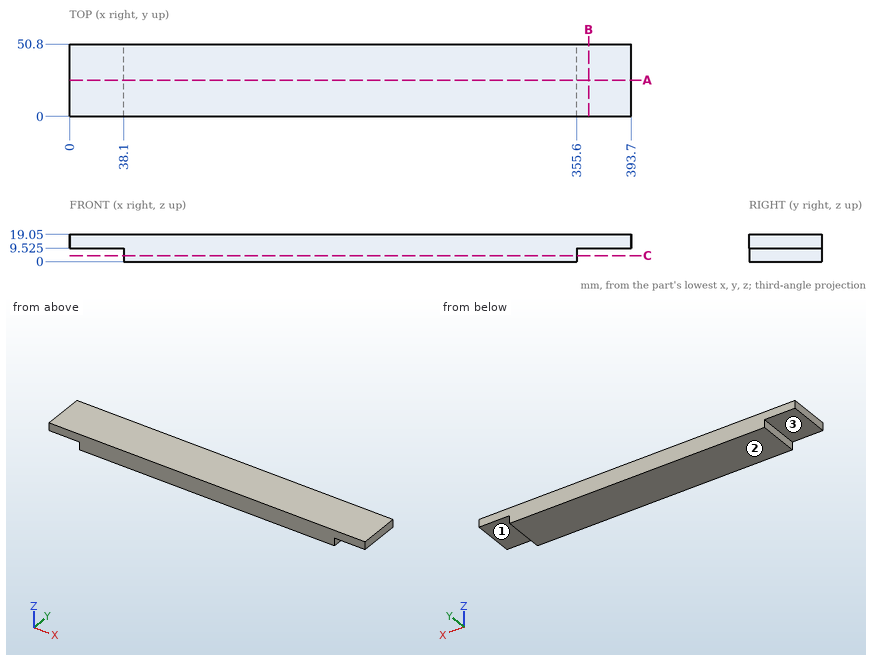
Print and shaded views of the part. All mm, measured from the part's lowest x, y and z. A direction names the side the tool comes from. Give positions to 0.01 mm unless a question says otherwise; leave off trailing zeros. Loops run counter-clockwise (first coordinate to the right, second up) from the corner with the lowest first, then second, coordinate; pieces in that order, holes last. Notation, with made-up numbers: (-1.5, -13) -> (10.5, -13) arc R18 ccw to (10.5, -3) -> close; hole circle Ø10 at (15.25, 77.25). An arc over 180 degrees is marked (long way). Use a Markdown table: item, result.
1. Which spindle directions (+Z, -Z, +X, -X, +Y, -Y) get a long thin tool onto all of the face, cutting with end or side? Do the marked faces 1, 2 and 3. Say none if no direction does.
Check result:
| item | result |
|---|---|
| face 1 | -Z, +X, +Y, -Y |
| face 2 | -Z, +X, -X, +Y, -Y |
| face 3 | -Z, -X, +Y, -Y |
2. Wall check: L1, parallel to X at y = 4, z = 2; L2, parallel to Z at x = 38, y = 6 (3 decimals). Give the ranges that are in metal, low to high. Write a range as [from, to].
Check result:
| item | result |
|---|---|
| L1 | x = [38.1, 355.6] |
| L2 | z = [9.525, 19.05] |
3. Flat gauge pins, fed straight in: pin 1 (10.5 mm diameter, centred on y = 13.5, z = 2.5, fed in from +X); pin 2 (19 mm diameter, centred on x = 23.5, y = 22.5, fed in from -Z) (3 decimals). Where does each tip first touch, or does it go through?
Check result:
| item | result |
|---|---|
| pin 1 | stops at x = 355.6 |
| pin 2 | stops at z = 9.525 |
4. Slice it at A-A (y = 25.5). List the corners of the cut face in (x, z) (3 decimals).
Check result:
| item | result |
|---|---|
| outline | (0, 9.525) -> (38.1, 9.525) -> (38.1, 0) -> (355.6, 0) -> (355.6, 9.525) -> (393.7, 9.525) -> (393.7, 19.05) -> (0, 19.05) -> close |
5. Slice it at B-B (x = 364). List the corners of the cut face in (y, z) (3 decimals).
Check result:
| item | result |
|---|---|
| outline | (0, 9.525) -> (50.8, 9.525) -> (50.8, 19.05) -> (0, 19.05) -> close |
6. Slice it at C-C (z = 4.25). List the corners of the cut face in (x, y), plus the area to 3 significant figures.
Check result:
| item | result |
|---|---|
| outline | (38.1, 0) -> (355.6, 0) -> (355.6, 50.8) -> (38.1, 50.8) -> close |
| area | 16,100 mm^2 |
